from build123d import *

# Parameters (mm, degrees)
EXTRUDE_1_DEPTH     = 2
SKETCH_3_W          = 2
SKETCH_3_H          = 4
EXTRUDE_2_DEPTH     = 2
SKETCH_4_W          = 16
SKETCH_4_H          = 3
CUT_EXTRUDE_1_DEPTH = 10
FILLET_1_R          = 1.5
SKETCH_5_R          = 1
CUT_EXTRUDE_2_DEPTH = 10
FILLET_2_R          = 1
FILLET_3_R          = 1.5


# Some blends are built 0.0001 mm under size
with BuildPart() as part:
    # 草图1 → 凸台-拉伸1 (new body)
    with BuildSketch(Plane(origin=(0, 0, 0), x_dir=(0, 0, -1), z_dir=(1, 0, 0))):
        Polygon((32, -10), (32, 0), (0, 0), (0, 5), (31.5, 5), (31.5, 8), (41, 8), (41, 5), (38, 5), (38, -10), align=None)
    extrude_1 = extrude(amount=EXTRUDE_1_DEPTH)

    # 草图3 → 凸台-拉伸2 (add)
    with BuildSketch(Plane(origin=(2, 0, 0), x_dir=(0, 0, -1), z_dir=(1, 0, 0))):
        with Locations((39, -8)):
            Rectangle(SKETCH_3_W, SKETCH_3_H)
    extrude_2 = extrude(amount=-EXTRUDE_2_DEPTH)

    # 镜向1: 凸台-拉伸1, 凸台-拉伸2 across plane
    add(extrude_1.mirror(Plane.XY))
    add(extrude_2.mirror(Plane.XY))

    # 草图4 → 切除-拉伸1 (cut)
    with BuildSketch(Plane(origin=(2, 0, 0), x_dir=(0, 0, -1), z_dir=(1, 0, 0))):
        Rectangle(SKETCH_4_W, SKETCH_4_H)
    extrude(amount=-CUT_EXTRUDE_1_DEPTH, mode=Mode.SUBTRACT)

    # 圆角1
    fillet_1_edges = [part.edges().sort_by_distance(p)[0] for p in [
        (1, 1.5, -8),
        (1, 1.5, 8),
    ]]
    fillet(fillet_1_edges, radius=FILLET_1_R - 0.0001)  # a hair under: the kernel refuses the full size

    # 草图5 → 切除-拉伸2 (cut)
    with BuildSketch(Plane(origin=(2, 0, 0), x_dir=(0, 0, -1), z_dir=(1, 0, 0))):
        with Locations((-38, 4)):
            Circle(SKETCH_5_R)
        with Locations((-38, -5)):
            Circle(SKETCH_5_R)
        with Locations((38, -5)):
            Circle(SKETCH_5_R)
        with Locations((38, 4)):
            Circle(SKETCH_5_R)
    extrude(amount=-CUT_EXTRUDE_2_DEPTH, mode=Mode.SUBTRACT)

    # 圆角2
    fillet_2_edges = [part.edges().sort_by_distance(p)[0] for p in [
        (1, 3, -38),
        (1, -4, -38),
        (1, -4, 38),
        (1, 3, 38),
    ]]
    fillet(fillet_2_edges, radius=FILLET_2_R)

    # 圆角3
    # the kernel refuses this fillet: 1.5 mm, written as the material it adds along each edge
    with BuildSketch(Plane(origin=(0, 0, 32), x_dir=(0, -1, 0), z_dir=(1, 0, 0)), Plane(origin=(0, 0, -32), x_dir=(0, 0, 1), z_dir=(1, 0, 0))) as fillet_3_piece_1:
        with BuildLine():
            CenterArc((FILLET_3_R, FILLET_3_R), FILLET_3_R, 180, 90)
            Line((0, FILLET_3_R), (0, 0))
            Line((0, 0), (FILLET_3_R, 0))
        make_face()
    extrude(amount=2)
    with BuildSketch(Plane(origin=(0, 5, -31.5), x_dir=(0, 0, 1), z_dir=(1, 0, 0)), Plane(origin=(0, 5, 31.5), x_dir=(0, 1, 0), z_dir=(1, 0, 0))) as fillet_3_piece_2:
        with BuildLine():
            CenterArc((FILLET_3_R, -FILLET_3_R), FILLET_3_R, 90, 90)
            Line((0, -FILLET_3_R), (0, 0))
            Line((0, 0), (FILLET_3_R, 0))
        make_face()
    extrude(amount=2)
    # the kernel refuses this fillet: 1.5 mm, written as the material it takes off along each edge
    with BuildSketch(Plane(origin=(-3.75, 8, -31.5), x_dir=(0, -1, 0), z_dir=(1, 0, 0)), Plane(origin=(-3.75, 8, 31.5), x_dir=(0, 0, 1), z_dir=(1, 0, 0))) as fillet_3_2_piece_1:
        with BuildLine():
            CenterArc((FILLET_3_R, FILLET_3_R), FILLET_3_R, 180, 90)
            Line((0, FILLET_3_R), (0, 0))
            Line((0, 0), (FILLET_3_R, 0))
        make_face()
    extrude(amount=9.5, mode=Mode.SUBTRACT)


solid = part.part
Geometry check sheet. Reference: the model listing, model coordinates, mm. A direction names the side the tool comes from. Coordinates: 2 decimals unless noted, no trailing zeros. Order: outer loops, then holes, each group sorted by start corner. A loop starts at its lowest first (then second) coordinate and runs counter-clockwise, first axis right, second up. Notation, with made-up numbers: (-28, -11.75) - (10, -11.75) arc R17 ccw to (10, -6.75) - close; hole circle Ø2 at (-6.5, 31.5). An arc over 180 degrees is marked (long way). Answer in a Markdown table with one row per item. Add a question column.
1) Cross-section at A-A, the plane y = -8.5. Record the cut outline in (x, z).
2) Gauge pin test, flat ends, axial feed: P1, Ø1, axis at x = 1.5, y = -0.5, coming from the +Z side; P2, Ø0.6, axis at x = 1.5, y = -8.5, coming from the +Z side; P3, Ø10, axis at y = 3.5, z = 8.5, coming from the -X side; P4, Ø1, axis at x = 0.5, z = 23, coming from the -Y side. Record the tip position at first contact, or that the pin passes through.
3) Material ranges on line 1 along Z through (x, y) = (0.7, -7.25); line 2 along Z through (x, y) = (1.35, 6.5); line 3 along Y through (x, z) = (1.9, 18.5), recorded low to high. Write a range as [from, to].
4) Release check for a two-part mould opening along Y. For faces 1 (the flat face through (1, -8, 40)), 2 (the flat face through (1, 0, -38)), 3 (the flat face through (1, 5, 0)) record: +Y half, -Y half, draft (parallel to the pull), parting line (faces both ways), or undercut.
5) Set-up check for faces 4 (the cylindrical face through (0.99, 1.05, 7.57)), 5 (the flat face through (1, 5, 40)), 6 (the flat face through (1, -6, -39)): record each of +Z, -Z, +X, -X, +Y, -Y from which the full face is reachable in a straight line by a thin tool's end or side.
6) Cross-section at C-C, the plane z = 1.5. Record the cut outline in (x, y), then the cut area to 3 significant figures.
7) Cross-section at B-B, the plane z = 26. Record the cut outline in (x, y), then the cut area to 3 significant figures.
Check result:
| question | item | result |
|---|---|---|
| 1 | outline | (0, -40) - (2, -40) - (2, -32) - (0, -32) - close; (0, 32) - (2, 32) - (2, 40) - (0, 40) - close |
| 2 | P1 | stops at z = 38 |
| 2 | P2 | stops at z = 40 |
| 2 | P3 | stops at x = 0 |
| 2 | P4 | stops at y = 0 |
| 3 | line 1 | z = [-40, -32], [32, 40] |
| 3 | line 2 | z = [-41, -31.5], [31.5, 41] |
| 3 | line 3 | y = [0, 5] |
| 4 | face 1 | draft |
| 4 | face 2 | undercut |
| 4 | face 3 | +Y half |
| 5 | face 4 | +X, -X, -Y |
| 5 | face 5 | +Z, +X, -X |
| 5 | face 6 | -Z, +X, -X |
| 6 | outline | (0, 1.5) - (2, 1.5) - (2, 5) - (0, 5) - close |
| 6 | area | 7.00 mm² |
| 7 | outline | (0, 0) - (2, 0) - (2, 5) - (0, 5) - close |
| 7 | area | 10.0 mm² |
